Part model, mm, in its own coordinate system. A direction names the side the tool comes from. Give positions to 0.01 mm unless a question says otherwise; leave off trailing zeros. Write each loop counter-clockwise with the first axis right and the second up, starting at its lowest first coordinate (ties: lowest second). Pieces come first, ordered by that corner, then holes. Notation, with made-up numbers: (-36, 28.25) - (-12, 28.25) arc R8 cw to (-12, 39.25) - close; hole circle Ø11 at (53, -23.75). An arc over 180 degrees is marked (long way). Answer in a Markdown table with one row per item. Add a question column.
1. Drop flat-ended pins along their axis: pin 1 Ø21.5 at (x, z) = (-12.5, -13) entering from -Y; pin 2 Ø6 at (y, z) = (41.5, -10) entering from +X; pin 3 Ø2 at (x, y) = (30, 43.5) entering from +Z. Give the stop position or say it passes through.
2. Band-saw the part on B-B on y = 7. Write the cut outline in (x, z).
3. Which spindle directions (+Z, -Z, +X, -X, +Y, -Y) get a long thin tool onto all of the face, cutting with end or side? Do faces 1 (the flat face through (31.42, 43.99, -10.21)), 2 (the flat face through (26.385, 49.014, -10.14)), 3 (the flat face through (1, 50, -1)). Say none if no direction does.
4. Pull direction Z, two halves, no side cores. Call faces 4 (the flat face through (1.673, 43.986, -9.79)), 5 (the cylindrical face through (44.617, 27.185, -5.858)), 6 (the flat face through (-16.877, 21.306, -36.457)): released by +Z, released by -Z, zero draft, split by the parting line, or undercut.
5. Band-saw the part on A-A on y = 34.5. Write the cut outline in (x, z), plus the area to 3 significant figures.
6. Probe line 1 along X through (y, z) = (36, 0); line 2 along Y through (x, z) = (29, 5.5); line 3 along Z through (x, y) = (-1, 23). List the from-to ranges inside material, lowest first.
7. Band-saw the part on C-C on y = 14. Write the cut outline in (x, z), plus the area to 3 significant figures.
```python
from build123d import *

# Parameters (mm, degrees)
SKETCH1_R                      = 45
BOSS_EXTRUDE1_DEPTH            = 50
CUT_EXTRUDE1_REACH             = 82.932
CUT_EXTRUDE1_DIRECTION_2_REACH = 82.932
FILLET1_R                      = 5
CUT_EXTRUDE2_DEPTH             = 2
SHELL1_START                   = 1.721637966
SHELL1_OUTLINE_R               = 40
SHELL1_DEPTH                   = 41.278362034
SHELL1_START_2                 = 43
SHELL1_2_OUTLINE_R             = 40
SHELL1_2_DEPTH                 = 2


with BuildPart() as part:
    # Sketch1 → Boss-Extrude1 (new body)
    with BuildSketch(Plane(origin=(0, 0, 0), x_dir=(1, 0, 0), z_dir=(0, 1, 0))):
        with Locations(Location((0, 0, 0), (0, 0, 270))):
            Circle(SKETCH1_R)
    extrude(amount=BOSS_EXTRUDE1_DEPTH)

    # Sketch2 → Cut-Extrude1 (cut, up to next)
    with BuildSketch(Plane.XY, mode=Mode.PRIVATE) as cut_extrude1_sk1:
        Polygon((45, 0), (-45, 0), (-45, 30.989485196), align=None)
    cut_extrude1_tool1 = extrude(cut_extrude1_sk1.sketch, amount=-CUT_EXTRUDE1_REACH, mode=Mode.PRIVATE) & part.part
    add(cut_extrude1_tool1.solids().sort_by_distance((-15, 10.329828, 0))[0], mode=Mode.SUBTRACT)

    # Sketch2 → Cut-Extrude1 direction 2 (cut, up to next)
    with BuildSketch(Plane.XY, mode=Mode.PRIVATE) as cut_extrude1_direction_2_sk1:
        Polygon((45, 0), (-45, 0), (-45, 30.989485196), align=None)
    cut_extrude1_direction_2_tool1 = extrude(cut_extrude1_direction_2_sk1.sketch, amount=CUT_EXTRUDE1_DIRECTION_2_REACH, mode=Mode.PRIVATE) & part.part
    add(cut_extrude1_direction_2_tool1.solids().sort_by_distance((-15, 10.329828, 0))[0], mode=Mode.SUBTRACT)

    # Fillet1
    fillet1_edges = [part.edges().sort_by_distance(p)[0] for p in [
        (0, 50, -45),
    ]]
    fillet(fillet1_edges, radius=FILLET1_R)

    # Sketch4 → Cut-Extrude2 (cut)
    with BuildSketch(Plane(origin=(0, 50, 0), x_dir=(1, 0, 0), z_dir=(0, 1, 0))):
        Polygon((-19.909733282, 20), (-18.114861487, 20), (-18.114861487, 2.051282051), (-10.422553795, 2.051282051), (-10.422553795, 0), (-19.909733282, 0), align=None)
        Polygon((5.423600051, 0), (8.06382441, 20), (8.320234666, 20), (16.577446205, 3.58974359), (24.814625692, 20), (25.075042359, 20), (27.731292359, 0), (25.928407743, 0), (24.013343641, 14.391025641), (16.793792359, 0), (16.389144923, 0), (9.141548769, 14.423076923), (7.230491077, 0), align=None)
    extrude(amount=-CUT_EXTRUDE2_DEPTH, mode=Mode.SUBTRACT)

    # Shell1: read off the stored shape, not the designer's step
    # Shell1 outline → Shell1 (cut)
    with BuildSketch(Plane(origin=(0, 0, 0), x_dir=(1, 0, 0), z_dir=(0, 1, 0)).offset(SHELL1_START)):
        Circle(SHELL1_OUTLINE_R)
    extrude(amount=SHELL1_DEPTH, mode=Mode.SUBTRACT)

    # Shell1 2 outline → Shell1 2 (cut)
    with BuildSketch(Plane(origin=(0, 0, 0), x_dir=(1, 0, 0), z_dir=(0, 1, 0)).offset(SHELL1_START_2)):
        Circle(SHELL1_2_OUTLINE_R)
        Polygon((-5.422553795, 7.051282051), (-5.422553795, -5), (-24.909733282, -5), (-24.909733282, 25), (-13.114861487, 25), (-13.114861487, 7.051282051), align=None, mode=Mode.SUBTRACT)
        Polygon((11.965201342, -2.331995426), (11.611690736, -5), (-0.279835267, -5), (3.680501271, 25), (11.401650362, 25), (16.572020474, 14.72448521), (21.729847234, 25), (29.454884993, 25), (33.439259993, -5), (21.549698117, -5), (21.1995112, -2.368469859), (19.879350477, -5), (13.30587364, -5), align=None, mode=Mode.SUBTRACT)
    extrude(amount=SHELL1_2_DEPTH, mode=Mode.SUBTRACT)


solid = part.part
```
Values:
| question | item | result |
|---|---|---|
| 1 | pin 1 | stops at y = 43 |
| 1 | pin 2 | stops at x = 44.45 |
| 1 | pin 3 | stops at z = 34.41 |
| 2 | outline | (24.67, -37.63) arc R45 ccw to (24.67, 37.63) - (24.67, 31.49) arc R40 cw to (24.67, -31.49) - close |
| 3 | face 1 | -Y |
| 3 | face 2 | +Y |
| 3 | face 3 | +Z, -Z, +X, -X, +Y |
| 4 | face 4 | undercut |
| 4 | face 5 | split by the parting line |
| 4 | face 6 | zero draft |
| 5 | outline | circle Ø90 at (0, 0); hole circle Ø80 at (0, 0) |
| 5 | area | 1,340 mm² |
| 6 | line 1 | x = -45 to -40, 40 to 45 |
| 6 | line 2 | y = 45 to 50 |
| 6 | line 3 | z = -44.99 to -39.99, 39.99 to 44.99 |
| 7 | outline | (4.34, -44.79) arc R45 ccw to (4.34, 44.79) - (4.34, 39.76) arc R40 cw to (4.34, -39.76) - close |
| 7 | area | 624 mm² |
